Design review of the part built by this model. Coordinates are the model's own, in mm. A direction names the side the tool comes from. Round coordinates to 2 decimals unless told otherwise and drop trailing zeros. Loops run counter-clockwise (first coordinate to the right, second up) from the corner with the lowest first, then second, coordinate; pieces in that order, holes last. Notation, with made-up numbers: (-13, 82.5) -> (12, 82.5) arc R9 ccw to (12, 99.5) -> close; hole circle Ø8 at (67.5, -26.75). An arc over 180 degrees is marked (long way). Answer as CSV lines item,"result". Start each with the question number.
```python
from build123d import *

# Parameters (mm, degrees)
SKETCH2_W         = 18.3
SKETCH2_H         = 2.8
SLOT_DEPTH        = 2.6
SKETCH3_W         = 1.98
SKETCH3_H         = 9.88
SKETCH4_W         = 0.99
SKETCH4_H         = 0.99
CIRPATTERN1_COUNT = 2
CIRPATTERN1_ANGLE = 90


with BuildPart() as part:
    # BodySke → Base-Revolve (revolve)
    with BuildSketch(Plane.XY):
        Polygon((0, 0), (0, 9.15), (0.85, 9.15), (5, 5), (40, 5), (40, 0), align=None)
    revolve(axis=Axis((-6.35, 0, 0), (1, 0, 0)))

    # Sketch2 → Slot (cut)
    with BuildSketch(Plane.ZY):
        Rectangle(SKETCH2_W, SKETCH2_H)
    extrude(amount=-SLOT_DEPTH, mode=Mode.SUBTRACT)

    # Sketch3 → Cross section 0
    with BuildSketch(Plane.ZY):
        Rectangle(SKETCH3_W, SKETCH3_H)
    # Sketch4 → Cross section 1
    with BuildSketch(Plane.ZY.offset(-5.98)):
        Rectangle(SKETCH4_W, SKETCH4_H)
    cross = loft(mode=Mode.SUBTRACT)

    # CirPattern1: Cross ×2 about axis
    cirpattern1_axis = Axis((0, 0, 0), (1, 0, 0))
    for i in range(1, CIRPATTERN1_COUNT):
        add(cross.rotate(cirpattern1_axis, i * CIRPATTERN1_ANGLE / (CIRPATTERN1_COUNT - 1)), mode=Mode.SUBTRACT)


solid = part.part
```
Q1. Mouldability with a two-part tool opening along Z and no side actions: class faces 1 (the flat face through (0, 5.3, 0.1)), 2 (the flat face through (5.98, 0, 0)), 3 (the conical face through (4.798, -1.128, -5.078)) as pulls with the +Z half, pulls with the -Z half, needs draft (parallel to the pull), parting line crosses it, or undercut.
Q2. To check wall thickness, follow probe 1 along Y at (x, z) = (5.5, 0.5); probe 2 along X at (y, z) = (5, -7.5); probe 3 along Z at (x, y) = (12, -0.75). State the ranges of each line that lie inside material, in increasing order. Write a range as from..to.
Q3. For pin 1 Ø1.1 at (y, z) = (0, 0) entering from -X; pin 2 Ø10 at (x, y) = (9.5, 5.5) entering from -Z; pin 3 Ø2 at (x, z) = (1.5, 5) entering from -Y, all flat-tipped, find the tip position at first contact; note any pin that passes through.
Q4. Machinability: for faces 4 (the flat face through (2.6, 0, -5)), 5 (the cylindrical face through (22.74, -1.08, -4.88)), 6 (the cylindrical face through (0.43, -9.15, 0.18)), which of the approach directions +Z, -Z, +X, -X, +Y, -Y give a long, thin tool a straight path to every point of the face, cutting with its end or side? Answer none if there is none.
Q5. Add section A-A, the plane x = 38.5. Give the boundary of the cut face in (y, z), and give its area (3 significant figures).
Worked answers:
1,face 1,"needs draft"
1,face 2,"undercut"
1,face 3,"parting line crosses it"
2,probe 1,"y = -4.97..-0.85, 0.85..4.97"
2,probe 2,"x = 0..0.99"
2,probe 3,"z = -4.94..4.94"
3,pin 1,"stops at x = 5.91"
3,pin 2,"stops at z = -4.97"
3,pin 3,"stops at y = -8.11"
4,face 4,"+Z, -Z, -X"
4,face 5,"+X"
4,face 6,"+X, -X, -Y"
5,outline,"circle Ø10 at (0, 0)"
5,area,"78.5 mm^2"
